Geometry check sheet. Reference: the model listing, model coordinates, mm. A direction names the side the tool comes from. Give positions to 0.01 mm unless a question says otherwise; leave off trailing zeros. Loops run counter-clockwise (first coordinate to the right, second up) from the corner with the lowest first, then second, coordinate; pieces in that order, holes last. Notation, with made-up numbers: (4.25, 35) -> (57.25, 35) arc R18 cw to (57.25, 53) -> close; hole circle Ø9 at (85.25, 66.5). An arc over 180 degrees is marked (long way). Write each question's results on one line, items separated by ' | '. Start each with the question number.
1) Depth check by flat-ended pin: pin 1 (5 mm diameter, centred on x = 487, z = 50, fed in from -Y); pin 2 (9.5 mm diameter, centred on x = 487, z = 1100, fed in from -Y); pin 3 (10 mm diameter, centred on x = 126, z = 449.5, fed in from -Y). Enter the tip coordinate at first touch or a pass-through.
2) Scan lines: line 1 (X direction, y = -1, z = 50); line 2 (X direction, y = -22.5, z = 764); line 3 (Z direction, x = 487, y = -2). Record each from-to range of solid material in increasing order. Write a range as from..to.
3) Set-up check for faces 1 (the face through (247, 0, 592)), 2 (the face through (0, -16, 592)): record each of +Z, -Z, +X, -X, +Y, -Y from which the full face is reachable in a straight line by a thin tool's end or side.
4) Sectioned sample at A-A on z = 935.5. Record the cut outline in (x, y), then the cut area to 3 significant figures.
5) Draft check along Y on faces 3 (the face through (487.675, -15.494, 1035.693)), 4 (the face through (487, -50, 592)), 5 (the face through (25, -25, 592)). Enter one of: pulls with the +Y half, pulls with the -Y half, needs draft (parallel to the pull), parting line crosses it, or undercut.
6) Sectioned sample at B-B on x = 248. Record the cut outline in (y, z), then the cut area to 3 significant figures.
```python
from build123d import *

# Parameters (mm, degrees)
SKETCH1_W                = 25
SKETCH1_H                = 50
SKETCH1_W_2              = 500
SKETCH1_H_2              = 18
BOSS_EXTRUDE1_DEPTH      = 1200
SKETCH2_R                = 15
CUT_EXTRUDE1_DEPTH       = 1
CUT_EXTRUDE1_DEPTH_BACK  = 501
F_6_0_6_DIAMETER_HOLE1_D = 6
LPATTERN1_COUNT          = 2
LPATTERN1_PITCH          = 50
LPATTERN1_COUNT_DIR2     = 2
LPATTERN1_PITCH_DIR2     = 474
LPATTERN2_COUNT          = 2
LPATTERN2_PITCH          = 1050
LPATTERN2_COPY_1_D       = 6
LPATTERN2_COPY_2_D       = 6
LPATTERN2_COPY_3_D       = 6


with BuildPart() as part:
    # Sketch1 → Boss-Extrude1 (new body)
    with BuildSketch(Plane.XY):
        with Locations((12.5, -25)):
            Rectangle(SKETCH1_W, SKETCH1_H)
        with Locations((250, 9)):
            Rectangle(SKETCH1_W_2, SKETCH1_H_2)
        with Locations((487.5, -25)):
            Rectangle(SKETCH1_W, SKETCH1_H)
    extrude(amount=BOSS_EXTRUDE1_DEPTH)

    # Sketch2 → Cut-Extrude1 (cut, two sides)
    with BuildSketch(Plane(origin=(500, 0, 0), x_dir=(0, 0, -1), z_dir=(1, 0, 0))) as cut_extrude1_sk:
        with Locations((-1050, -20)):
            Circle(SKETCH2_R)
        with Locations((-150, -20)):
            Circle(SKETCH2_R)
    extrude(amount=CUT_EXTRUDE1_DEPTH, mode=Mode.SUBTRACT)
    extrude(cut_extrude1_sk.sketch, amount=-CUT_EXTRUDE1_DEPTH_BACK, mode=Mode.SUBTRACT)

    # Ø6.0 (6) Diameter Hole1 (through all)
    with Locations(Plane(origin=(0, 18, 0), x_dir=(1, 0, 0), z_dir=(0, 1, 0))):
        with Locations((13, -1150)):
            f_6_0_6_diameter_hole1 = Hole(F_6_0_6_DIAMETER_HOLE1_D / 2)

    # LPattern1: 6.0 _6_ Diameter Hole1 2 × 2
    with Locations(*[(j * LPATTERN1_PITCH_DIR2, 0, -i * LPATTERN1_PITCH) for i in range(LPATTERN1_COUNT) for j in range(LPATTERN1_COUNT_DIR2) if (i, j) != (0, 0)]):
        add(f_6_0_6_diameter_hole1, mode=Mode.SUBTRACT)

    # LPattern2: Ø6.0 (6) Diameter Hole1 ×2
    with Locations(*[(0, 0, -i * LPATTERN2_PITCH) for i in range(1, LPATTERN2_COUNT)]):
        add(f_6_0_6_diameter_hole1, mode=Mode.SUBTRACT)

    # LPattern2 copy 1 (through all)
    with Locations(Plane(origin=(474, 18, -1050), x_dir=(1, 0, 0), z_dir=(0, 1, 0))):
        with Locations((13, -1150)):
            Hole(LPATTERN2_COPY_1_D / 2)

    # LPattern2 copy 2 (through all)
    with Locations(Plane(origin=(0, 18, -1100), x_dir=(1, 0, 0), z_dir=(0, 1, 0))):
        with Locations((13, -1150)):
            Hole(LPATTERN2_COPY_2_D / 2)

    # LPattern2 copy 3 (through all)
    with Locations(Plane(origin=(474, 18, -1100), x_dir=(1, 0, 0), z_dir=(0, 1, 0))):
        with Locations((13, -1150)):
            Hole(LPATTERN2_COPY_3_D / 2)


solid = part.part
```
Result:
1) pin 1: through | pin 2: y = -50 | pin 3: y = 0
2) line 1: 0..10, 16..25, 475..484, 490..500 | line 2: 0..25, 475..500 | line 3: 0..47, 53..97, 103..1097, 1103..1147, 1153..1200
3) face 1: +Z, -Z, -Y | face 2: +Z, -Z, -X, +Y, -Y
4) outline: (0, -50) -> (25, -50) -> (25, 0) -> (475, 0) -> (475, -50) -> (500, -50) -> (500, 18) -> (0, 18) -> close | area: 11,500 mm^2
5) face 3: undercut | face 4: pulls with the -Y half | face 5: needs draft
6) outline: (0, 0) -> (18, 0) -> (18, 1200) -> (0, 1200) -> close | area: 21,600 mm^2
